Here's how the part is built. I have some questions about the finished solid (model axes, mm). A direction names the side the tool comes from. Coordinates: 2 decimals unless noted, no trailing zeros. Order: outer loops, then holes, each group sorted by start corner. A loop starts at its lowest first (then second) coordinate and runs counter-clockwise, first axis right, second up. Notation, with made-up numbers: M 81.5,-2.5 L 87.5,-2.5 A17 cw 87.5,19.5 Z; hole C -39.5,63.25 d5. An arc over 180 degrees is marked long. Answer as CSV lines item,"result". Start each with the question number.
```python
from build123d import *

# Parameters (mm, degrees)
SKETCH1_R       = 5.270407467
FEATURE_A_DEPTH = 38.1
SKETCH2_W       = 10.540814934
SKETCH2_H       = 25.4
FEATURE_B_DEPTH = 1.246819584
SKETCH5_W       = 63.5
SKETCH5_H       = 4.173585558
FEATURE_C_DEPTH = 10.027755954
SKETCH6_W       = 0.800228097
SKETCH6_H       = 38.0746
FEATURE_D_DEPTH = 4.064
SKETCH7_W       = 25.37968
SKETCH7_H       = 3.975694803
SKETCH7_H_2     = 4.064
FEATURE_E_DEPTH = 0.800228097


with BuildPart() as part:
    # Sketch1 → Feature A (new body)
    with BuildSketch(Plane.XY):
        Circle(SKETCH1_R)
    extrude(amount=-FEATURE_A_DEPTH)

    # Sketch2 → Feature B (add)
    with BuildSketch(Plane(origin=(0, 0, -38.1), x_dir=(-1, 0, 0), z_dir=(0, 0, -1))):
        with Locations((0, 12.7)):
            Rectangle(SKETCH2_W, SKETCH2_H)
    extrude(amount=-FEATURE_B_DEPTH)

    # Sketch5 → Feature C (add)
    with BuildSketch(Plane(origin=(0, 25.4, 0), x_dir=(1, 0, 0), z_dir=(0, 1, 0))):
        with Locations((0, 37.71392)):
            Rectangle(SKETCH5_W, SKETCH5_H)
    extrude(amount=FEATURE_C_DEPTH)

    # Sketch6 → Feature D (add)
    with BuildSketch(Plane.XY.offset(-35.627127221)):
        with Locations((-32.150114049, 44.4373)):
            Rectangle(SKETCH6_W, SKETCH6_H)
        with Locations((32.150114049, 44.4373)):
            Rectangle(SKETCH6_W, SKETCH6_H)
    extrude(amount=-FEATURE_D_DEPTH)

    # Sketch7 → Feature E (add)
    with BuildSketch(Plane(origin=(0, 63.4746, 0), x_dir=(1, 0, 0), z_dir=(0, 1, 0))):
        with Locations((-19.860388097, 37.614974623)):
            Rectangle(SKETCH7_W, SKETCH7_H)
        with Locations((19.860388097, 37.659127221)):
            Rectangle(SKETCH7_W, SKETCH7_H_2)
    extrude(amount=FEATURE_E_DEPTH)


solid = part.part
```
1) Suppose I cut it at D-D on z = -23. Please give me the cut outline in (x, y).
2) Will these pins go through, and if not, where does the flat tip stop? pin 1 Ø1.2 at (x, z) = (21, -36.5) entering from -Y; pin 2 Ø5.5 at (x, y) = (1, 6.5) entering from -Z; pin 3 Ø8 at (x, z) = (21.5, -28.5) entering from -Y; pin 4 Ø1 at (y, z) = (9.5, -37) entering from -X.
3) If we mould it in two halves opening along Y, with no side actions, what happens to faces 1 (the face through (-20, 64.275, -38)), 2 (the face through (-32.55, 45, -38)), 3 (the face through (-31.75, 49, -38))? For each: released by +Y, released by -Y, zero draft, split by the parting line, or undercut.
4) Suppose I cut it at C-C on x = 0. Please give me the cut outline in (y, z), plus the area to 3 significant figures.
5) Suppose I cut it at B-B on y = 55. Please give me the cut outline in (x, z).
6) Which directions (+Z, -Z, +X, -X, +Y, -Y) give clear straight access to the entire face, cutting with the end or side of a thin tool? Please do faces 4 (the face through (5.03, 1.58, -18.78)), 5 (the face through (0, 29, -35.627)), 6 (the face through (19, 63.475, -38)), 7 (the face through (32, 54, -39.691)), 8 (the face through (0, 10, -38.1)).
7) Suppose I cut it at A-A on x = -14. Please give me the cut outline in (y, z).
8) I need wall thicknesses on line 1 (Y direction, x = 21.5, z = -36); line 2 (Z direction, x = -4, y = 15.5); line 3 (Z direction, x = -22.5, y = 28). Which ranges of each line are inside material? Lowest first, please. Write a range as [from, to].
Output:
1,outline,"C 0,0 d10.54"
2,pin 1,"y = 25.4"
2,pin 2,"z = -38.1"
2,pin 3,"through"
2,pin 4,"x = -5.27"
3,face 1,"released by +Y"
3,face 2,"zero draft"
3,face 3,"undercut"
4,outline,"M -5.27,-38.1 L 25.4,-38.1 L 25.4,-39.8 L 35.43,-39.8 L 35.43,-35.63 L 25.4,-35.63 L 25.4,-36.85 L 5.27,-36.85 L 5.27,0 L -5.27,0 Z"
4,area,"469 mm²"
5,outline,"M -32.55,-39.69 L -31.75,-39.69 L -31.75,-35.63 L -32.55,-35.63 Z; M 31.75,-39.69 L 32.55,-39.69 L 32.55,-35.63 L 31.75,-35.63 Z"
6,face 4,"+Z"
6,face 5,"+Z, +X, -X, +Y"
6,face 6,"+Z, -Z"
6,face 7,"-Z, +X, +Y"
6,face 8,"-Z, +X, -X, -Y"
7,outline,"M 25.4,-39.8 L 35.43,-39.8 L 35.43,-35.63 L 25.4,-35.63 Z; M 63.47,-39.6 L 64.27,-39.6 L 64.27,-35.63 L 63.47,-35.63 Z"
8,line 1,"[25.4, 35.43], [63.47, 64.27]"
8,line 2,"[-38.1, -36.85]"
8,line 3,"[-39.8, -35.63]"
